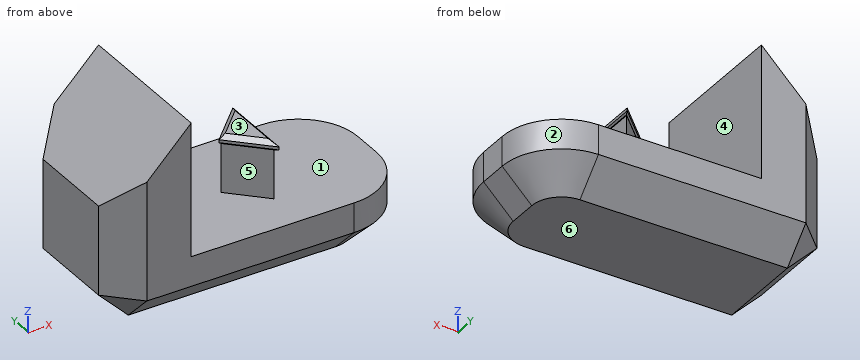
from build123d import *

# Parameters (mm, degrees)
PAD_DEPTH       = 10
PAD001_DEPTH    = 3.3
PAD002_DEPTH    = 0.6
CHAMFER004_SIZE = 0.1
CHAMFER005_SIZE = 0.3
FILLET_R        = 4
CHAMFER_SIZE    = 2


with BuildPart() as part:
    # Sketch → Pad (new body)
    with BuildSketch(Plane.XZ):
        Polygon((0, 8), (0, 0), (20, 0), (20, 4), (5, 4), (5, 13), align=None)
    extrude(amount=PAD_DEPTH)

    # Sketch001 → Pad001 (new body)
    with BuildSketch(Plane(origin=(0, 0, 4), x_dir=(-1, 0, 0), z_dir=(0, 0, 1))):
        Polygon((-12.35, 7.2), (-12.35, 2.8), (-10.15, 5), align=None)
    extrude(amount=PAD001_DEPTH)

    # Sketch003 → Pad002 (new body)
    with BuildSketch(Plane(origin=(0, 0, 7.3), x_dir=(-1, 0, 0), z_dir=(0, 0, 1))):
        Polygon((-12.5, 2.5), (-10, 5), (-12.5, 7.5), align=None)
    extrude(amount=PAD002_DEPTH)

    # Chamfer004
    chamfer004_edges = [part.edges().sort_by_distance(p)[0] for p in [
        (12.5, -5, 7.3),
        (11.25, -6.25, 7.3),
        (11.25, -3.75, 7.3),
    ]]
    chamfer(chamfer004_edges, length=CHAMFER004_SIZE)

    # Chamfer005
    chamfer005_edges = [part.edges().sort_by_distance(p)[0] for p in [
        (12.5, -5, 7.9),
        (11.25, -3.75, 7.9),
        (11.25, -6.25, 7.9),
    ]]
    chamfer(chamfer005_edges, length=CHAMFER005_SIZE)

    # Fillet
    fillet_edges = [part.edges().sort_by_distance(p)[0] for p in [
        (20, 0, 2),
        (20, -10, 2),
    ]]
    fillet(fillet_edges, radius=FILLET_R)

    # Chamfer
    chamfer_edges = [part.edges().sort_by_distance(p)[0] for p in [
        (8, 0, 0),
        (18.828427, -1.171573, 0),
        (20, -5, 0),
        (18.828427, -8.828427, 0),
        (8, -10, 0),
        (0, -5, 0),
        (0, 0, 4),
        (0, -10, 4),
    ]]
    chamfer(chamfer_edges, length=CHAMFER_SIZE)


solid = part.part
Source: CAD feature listing. Evaluate the final solid. Frame: model axes, mm. Face numbers are marked on the shaded views. A direction names the side the tool comes from. Give positions to 0.01 mm unless a question says otherwise; leave off trailing zeros. Write each loop counter-clockwise with the first axis right and the second up, starting at its lowest first coordinate (ties: lowest second). Pieces come first, ordered by that corner, then holes. Notation, with made-up numbers: (67.5, 57.5) - (92.5, 57.5) arc R8 cw to (92.5, 64.5) - close; hole circle Ø8 at (20.5, 83). An arc over 180 degrees is marked (long way). Write item = value, one per line. Start each with the question number.
Q1. Cut plane B-B, the plane z = 3.25. Return loops of the section in (x, y).
Q2. Reachability of the marked faces 4, 5 and 6 from +Z, -Z, +X, -X, +Y, -Y: full face, straight path, thin tool, end or side. Return the list, or none.
Q3. Cut plane C-C, the plane x = 15.5. Return loops of the section in (y, z), then the cut area to 3 significant figures.
Q4. Draft query along X for the marked faces 1, 2 and 3. Return one class per face: +X half, -X half, draft (parallel to the pull), parting line (faces both ways), or undercut.
Q5. Material intervals for probe 1 along Z at (x, y) = (8.25, -5.5); probe 2 along Y at (x, z) = (9.25, 1); probe 3 along Y at (x, z) = (10.5, 5.25), sorted ascending.
Q6. Pin query (flat end, axial travel): pin 1 Ø5 at (y, z) = (-4, 10.5) entering from +X; pin 2 Ø1.5 at (x, y) = (16.5, -8) entering from +Z; pin 3 Ø2 at (x, y) = (11, -5.5) entering from +Z. Return the tip coordinate at first contact, or that it passes through.
Q7. Cut plane A-A, the plane z = 5.5. Return loops of the section in (x, y), then the cut area to 3 significant figures.
Computed values:
q1.outline = (0, -8) - (2, -10) - (16, -10) arc R4 ccw to (20, -6) - (20, -4) arc R4 ccw to (16, 0) - (2, 0) - (0, -2) - close
q2.face_4 = +Z, +Y, -Y
q2.face_5 = -Y
q2.face_6 = -Z, +X, -X, +Y, -Y
q3.outline = (-10, 2) - (-8, 0) - (-2, 0) - (0, 2) - (0, 4) - (-10, 4) - close
q3.area = 36.0 mm²
q4.face_1 = undercut
q4.face_2 = +X half
q4.face_3 = draft
q5.probe_1 = 0 to 4
q5.probe_2 = -9 to -1
q5.probe_3 = -5.35 to -4.65
q6.pin_1 = 5
q6.pin_2 = 4
q6.pin_3 = 7.9
q7.outline = (0, -8) - (2, -10) - (5, -10) - (5, 0) - (2, 0) - (0, -2) - close; (10.15, -5) - (12.35, -7.2) - (12.35, -2.8) - close
q7.area = 50.8 mm²
